from build123d import *

# Parameters (mm, degrees)
SKETCH_1_W          = 1440
SKETCH_1_H          = 1410
EXTRUDE_1_DEPTH     = 750
SKETCH_2_W          = 690
SKETCH_2_H          = 1440
CUT_EXTRUDE_1_DEPTH = 2251
SKETCH_3_W          = 1440
SKETCH_3_H          = 690
CUT_EXTRUDE_2_DEPTH = 2241.027901612
SKETCH_4_W          = 24
SKETCH_4_H          = 24
CUT_EXTRUDE_3_DEPTH = 2251


with BuildPart() as part:
    # Эскиз1 → Бобышка-Вытянуть1 (new body)
    with BuildSketch(Plane.XY):
        Polygon((30, 1500), (30, 1485), (1470, 1485), (1470, 1500), (1500, 1500), (1500, 0), (1470, 0), (1470, 15), (30, 15), (30, 0), (0, 0), (0, 1500), align=None)
        with Locations((750, 750)):
            Rectangle(SKETCH_1_W, SKETCH_1_H, mode=Mode.SUBTRACT)
    extrude(amount=EXTRUDE_1_DEPTH)

    # Эскиз2 → Вырез-Вытянуть1 (cut, through all)
    with BuildSketch(Plane(origin=(1500, 0, 0), x_dir=(0, 0, -1), z_dir=(1, 0, 0))):
        with Locations((-375, 750)):
            Rectangle(SKETCH_2_W, SKETCH_2_H)
    extrude(amount=-CUT_EXTRUDE_1_DEPTH, mode=Mode.SUBTRACT)

    # Эскиз3 → Вырез-Вытянуть2 (cut, through all)
    with BuildSketch(Plane(origin=(0, 1485, 0), x_dir=(1, 0, 0), z_dir=(0, 1, 0))):
        with Locations((750, -375)):
            Rectangle(SKETCH_3_W, SKETCH_3_H)
    extrude(amount=-CUT_EXTRUDE_2_DEPTH, mode=Mode.SUBTRACT)

    # Эскиз4 → Вырез-Вытянуть3 (cut, through all)
    with BuildSketch(Plane(origin=(0, 1500, 0), x_dir=(1, 0, 0), z_dir=(0, 1, 0))):
        with Locations((15, -15)):
            Rectangle(SKETCH_4_W, SKETCH_4_H)
        with Locations((1485, -735)):
            Rectangle(SKETCH_4_W, SKETCH_4_H)
        with Locations((1485, -15)):
            Rectangle(SKETCH_4_W, SKETCH_4_H)
        with Locations((15, -735)):
            Rectangle(SKETCH_4_W, SKETCH_4_H)
    extrude(amount=-CUT_EXTRUDE_3_DEPTH, mode=Mode.SUBTRACT)


solid = part.part
Check sheet for the modelled part. Datum: model origin and axes. Units: mm. Round coordinates to 2 decimals unless told otherwise and drop trailing zeros. Loops run counter-clockwise (first coordinate to the right, second up) from the corner with the lowest first, then second, coordinate; pieces in that order, holes last. Notation, with made-up numbers: (46, 0.5) -> (68, 0.5) arc R22 ccw to (68, 10.5) -> close; hole circle Ø6 at (86, 77). An arc over 180 degrees is marked (long way). Put each result on its own line as item: value. Start each with the question number.
1. Gauge pin test, flat end, axial feed: pin 1 (9 mm diameter, centred on x = 660, z = 19.5, fed in from +Y). Record the tip position at first contact, or that the pin passes through.
2. Section check B-B (z = 621.5). Enter the section's corners in (x, y).
3. Draft check along Y on faces 1 (the face through (1500, 976, 734)), 2 (the face through (413, 1461, 30)). Enter one of: +Y half, -Y half, draft (parallel to the pull), parting line (faces both ways), or undercut.
4. Section check C-C (x = 248). Enter the section's corners in (y, z).
5. Section check A-A (y = 894.5). Give the number of separate pieces and of enclosed holes in the cut face, plus the area to 3 significant figures.
Findings:
1. pin 1: stops at y = 1485
2. outline: (0, 0) -> (30, 0) -> (30, 30) -> (0, 30) -> close; (0, 1470) -> (30, 1470) -> (30, 1500) -> (0, 1500) -> close; (1470, 0) -> (1500, 0) -> (1500, 30) -> (1470, 30) -> close; (1470, 1470) -> (1500, 1470) -> (1500, 1500) -> (1470, 1500) -> close
3. face 1: draft
3. face 2: undercut
4. outline: (15, 0) -> (45, 0) -> (45, 30) -> (15, 30) -> close; (15, 720) -> (45, 720) -> (45, 750) -> (15, 750) -> close; (1455, 0) -> (1485, 0) -> (1485, 30) -> (1455, 30) -> close; (1455, 720) -> (1485, 720) -> (1485, 750) -> (1455, 750) -> close
5. separate pieces: 4
5. enclosed holes: 4
5. area: 1,300 mm^2
